The listing builds one solid part. Answer for the finished solid, in the listing's coordinates (mm). Face numbers are marked on the shaded views. Round coordinates to 2 decimals unless told otherwise and drop trailing zeros. Write each loop counter-clockwise with the first axis right and the second up, starting at its lowest first coordinate (ties: lowest second). Pieces come first, ordered by that corner, then holes. Notation, with made-up numbers: M 2,53.25 L 39,53.25 A12 cw 39,62.25 Z; hole C 49,22.5 d6. An arc over 180 degrees is marked long. Write each question's results on one line, items separated by ' | '.
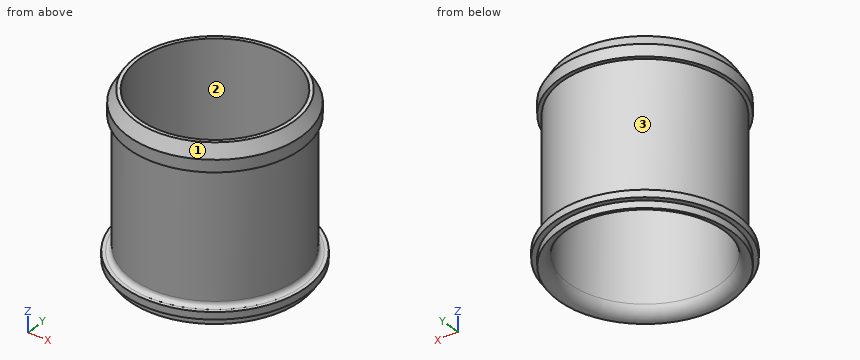
from build123d import *

# Parameters (mm, degrees)
F2_SIZE2 = 3
F2_SIZE  = 5
F3_R     = 2


# Not quite as in the source:
# - a fillet or chamfer that OpenCascade refuses, or shapes differently, is made with other operations: its cross-section is extruded or revolved along the edge and cut away or added


with BuildPart() as f1:
    # F0 (on Front) → F1 (revolve)
    with BuildSketch(Plane.XZ):
        Polygon((34.5, 70), (31.5, 70), (31.5, 0), (36, 0), (36, 3), (38, 3), (38, 6), (34.5, 6), (34.5, 60), (36, 60), (36, 70), align=None)
    revolve(axis=Axis((0, 0, 35), (0, 0, 1)))

    # F2
    f2_edges = [f1.edges().sort_by_distance(p)[0] for p in [
        (-36, 0, 70),
    ]]
    f2_side = f1.faces().sort_by_distance((-36, 0, 65))[0]
    chamfer(f2_edges, length=F2_SIZE, length2=F2_SIZE2, reference=f2_side)

    # F3
    f3_edges = [f1.edges().sort_by_distance(p)[0] for p in [
        (-34.5, 0, 6),
    ]]
    fillet(f3_edges, radius=F3_R)

    # F4: fillet of radius 5 on 1 edges, made by hand

    # F4_s1 → F4_t2 (revolve, cut)
    with BuildSketch(Plane.XZ):
        with BuildLine():
            ThreePointArc((31.5, 4.9749371855), (32.7919007565, 1.6208352193), (36, 0))
            Line((36, 0), (31.5, 0))
            Line((31.5, 0), (31.5, 4.9749371855))
        make_face()
    revolve(axis=Axis((0, 0, 0), (0, 0, 1)), mode=Mode.SUBTRACT)


solid = f1.part
1) Section A-A (y = 0) is taken. Determine the outline of the cut face in (x, z), then the cut area to 3 significant figures.
Return value:
outline: M -38,3 L -36,3 L -36,0 A5 ccw -31.5,4.97 L -31.5,70 L -33,70 L -36,65 L -36,60 L -34.5,60 L -34.5,8 A2 cw -36.5,6 L -38,6 Z; M 31.5,4.97 A5 ccw 36,0 L 36,3 L 38,3 L 38,6 L 36.5,6 A2 cw 34.5,8 L 34.5,60 L 36,60 L 36,65 L 33,70 L 31.5,70 Z | area: 456 mm²
2) Section C-C (z = 32.5) is taken. Determine the outline of the cut face in (x, y).
Return value:
outline: C 0,0 d69; hole C 0,0 d63
3) Each of these flat-tipped pins is pushed along its axis until it touches: pin 1 (6 mm diameter, centred on x = 28, z = 62.5, fed in from -Y); pin 2 (8 mm diameter, centred on y = 27, z = 23.5, fed in from +X); pin 3 (5 mm diameter, centred on y = 21.5, z = 61.5, fed in from +X). Where does it stop, or does it pass through?
Return value:
pin 1: y = -25.9 | pin 2: x = 25.71 | pin 3: x = 30.58
4) Find the intervals of material crossed by line 1 (Y direction, x = 0, z = 37); line 2 (Y direction, x = -14, z = 18); line 3 (X direction, y = 26.5, z = 53.5), in increasing order.
Return value:
line 1: -34.5 to -31.5, 31.5 to 34.5 | line 2: -31.53 to -28.22, 28.22 to 31.53 | line 3: -22.09 to -17.03, 17.03 to 22.09
5) The mould has two halves that part along Z. Classify the marked faces 1, 2 and 3: +Z half, -Z half, draft (parallel to the pull), parting line (faces both ways), or undercut.
Return value:
face 1: +Z half | face 2: draft | face 3: undercut
